CAD build for the part. Positions are in the model's coordinates, mm. Coordinates: 2 decimals unless noted, no trailing zeros. Loops run counter-clockwise (first coordinate to the right, second up) from the corner with the lowest first, then second, coordinate; pieces in that order, holes last.
1) Saw through at C-C, the plane x = 48.5. Write the cut outline in (y, z), and give its area (3 significant figures).
2) Pin check, flat tips, straight feed: pin 1 Ø10 at (x, z) = (27.5, 28) entering from +Y; pin 2 Ø1.5 at (y, z) = (-22.5, 25.5) entering from +X; pin 3 Ø2 at (x, y) = (18, -24.5) entering from +Z. Stop position of each tip, or through.
3) Saw through at A-A, the plane y = -25. Write the cut outline in (x, z).
4) Saw through at B-B, the plane z = 21. Write the cut outline in (x, y), and give its area (3 significant figures).
5) Wall check: line 1 along Z through (x, y) = (9.5, -15.5); line 2 along Z through (x, y) = (23, -32); line 3 along X through (y, z) = (-4.5, 28). Give the ranges that are in metal, low to high.
```python
from build123d import *

# Parameters (mm, degrees)
F1_DEPTH = 38.1
F3_DEPTH = 38.1
F5_DEPTH = 38.1


with BuildPart() as f1:
    # F0 (on Front) → F1 (new body)
    with BuildSketch(Plane.XZ):
        Polygon((57.148678, 38.1), (0, 37.711234), (0, 0), (57.148678, 0), align=None)
    extrude(amount=F1_DEPTH)

    # F2 (on face) → F3 (cut)
    with BuildSketch(Plane.XZ.offset(38.1)):
        with BuildLine():
            ThreePointArc((0, 27.63082), (3.777567, 34.45559), (10.83186, 37.78492))
            Line((10.83186, 37.78492), (0, 37.711234))
            Line((0, 37.711234), (0, 27.63082))
        make_face()
    extrude(amount=-F3_DEPTH, mode=Mode.SUBTRACT)

    # F4 (on face) → F5 (cut)
    with BuildSketch(Plane.XZ.offset(38.1)):
        with BuildLine():
            Line((57.148678, 38.1), (33.990269, 37.94246))
            ThreePointArc((33.990269, 37.94246), (42.496702, 24.729622), (57.148678, 19.05))
            Line((57.148678, 19.05), (57.148678, 38.1))
        make_face()
    extrude(amount=-F5_DEPTH, mode=Mode.SUBTRACT)


solid = f1.part
```
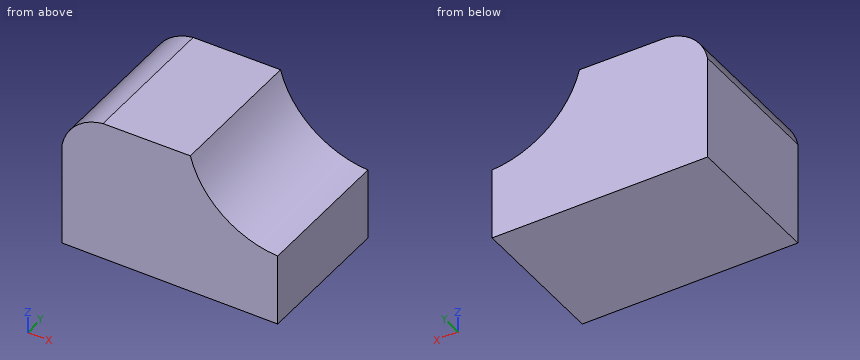
Data:
1. outline: (-38.1, 0) - (0, 0) - (0, 21.09) - (-38.1, 21.09) - close
1. area: 803 mm2
2. pin 1: stops at y = 0
2. pin 2: stops at x = 42.47
2. pin 3: stops at z = 37.84
3. outline: (0, 0) - (57.15, 0) - (57.15, 19.05) arc R25.4 cw to (33.99, 37.94) - (10.83, 37.78) arc R12.7 ccw to (0, 27.63) - close
4. outline: (0, -38.1) - (48.7, -38.1) - (48.7, 0) - (0, 0) - close
4. area: 1,860 mm2
5. line 1: z = 0 to 37.54
5. line 2: z = 0 to 37.87
5. line 3: x = 0.08 to 39.17
